Model file for the job. Use its own axes, mm. Face numbers are marked on the shaded views. A direction names the side the tool comes from. Round coordinates to 2 decimals unless told otherwise and drop trailing zeros. Loops run counter-clockwise (first coordinate to the right, second up) from the corner with the lowest first, then second, coordinate; pieces in that order, holes last. Notation, with made-up numbers: M -38.5,-22.75 L -27.5,-22.75 A32 cw -27.5,13.25 Z; hole C 87.5,40 d3. An arc over 180 degrees is marked long. Answer in a Markdown table with one row per item.
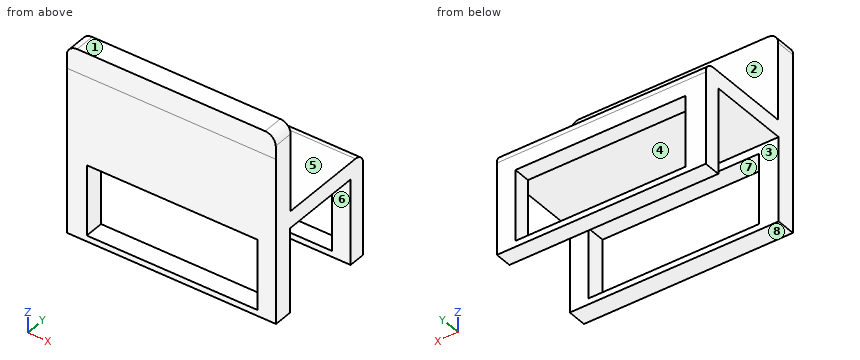
from build123d import *

# Parameters (mm, degrees)
F1_DEPTH = 101.6
F2_R     = 5.08
F4_W     = 83.005025
F4_H     = 34.228876
F5_DEPTH = 25.4
F3_W     = 82.719785
F3_H     = 34.51412
F6_DEPTH = 25.4


with BuildPart() as f1:
    # F0 (on Right) → F1 (new body)
    with BuildSketch(Plane.YZ):
        Polygon((-64.356416, 42.612657), (-64.071178, 30.91779), (-64.071178, -49.234834), (-54.658234, -49.234834), (-54.658234, -8.160179), (-14.724543, -8.160179), (-14.724543, -49.805317), (-6.452564, -49.805317), (-6.452564, -7.589698), (-6.452564, 0), (-54.372992, 0), (-54.372992, 42.612657), align=None)
    extrude(amount=F1_DEPTH)

    # F2
    f2_edges = [f1.edges().sort_by_distance(p)[0] for p in [
        (101.6, -59.364704, 42.612657),
        (0, -59.364704, 42.612657),
        (50.8, -6.452564, 0),
    ]]
    fillet(f2_edges, radius=F2_R)

    # F4 (on face) → F5 (cut)
    with BuildSketch(Plane.XZ.offset(64.071178)):
        with Locations((51.064864, -29.237166)):
            Rectangle(F4_W, F4_H)
    extrude(amount=-F5_DEPTH, mode=Mode.SUBTRACT)

    # F3 (on face) → F6 (cut)
    with BuildSketch(Plane(origin=(0, -6.452564, 0), x_dir=(-1, 0, 0), z_dir=(0, 1, 0))):
        with Locations((-51.207484, -29.665028)):
            Rectangle(F3_W, F3_H)
    extrude(amount=-F6_DEPTH, mode=Mode.SUBTRACT)


solid = f1.part
1. Saw through at A-A (x = 62). Write the cut outline in (y, z), and give its area (3 significant figures).
Verdict:
| item | result |
|---|---|
| outline | M -64.36,42.61 L -64.07,30.92 L -64.07,-12.12 L -54.66,-12.12 L -54.66,-8.16 L -14.72,-8.16 L -14.72,-12.41 L -6.45,-12.41 L -6.45,-5.08 A5.08 ccw -11.53,0 L -54.37,0 L -54.37,42.61 Z; M -64.07,-49.23 L -54.66,-49.23 L -54.66,-46.35 L -64.07,-46.35 Z; M -14.72,-49.81 L -6.45,-49.81 L -6.45,-46.92 L -14.72,-46.92 Z |
| area | 1,000 mm² |
2. Saw through at D-D (y = -13.5). Write the cut outline in (x, z), and give its area (3 significant figures).
Verdict:
| item | result |
|---|---|
| outline | M 0,-49.81 L 101.6,-49.81 L 101.6,0 L 0,0 Z; hole M 9.85,-46.92 L 92.57,-46.92 L 92.57,-12.41 L 9.85,-12.41 Z |
| area | 2,210 mm² |
3. Saw through at B-B (z = -30.5). Write the cut outline in (x, y), and give its area (3 significant figures).
Verdict:
| item | result |
|---|---|
| outline | M 0,-64.07 L 9.56,-64.07 L 9.56,-54.66 L 0,-54.66 Z; M 0,-14.72 L 9.85,-14.72 L 9.85,-6.45 L 0,-6.45 Z; M 92.57,-64.07 L 101.6,-64.07 L 101.6,-54.66 L 92.57,-54.66 Z; M 92.57,-14.72 L 101.6,-14.72 L 101.6,-6.45 L 92.57,-6.45 Z |
| area | 331 mm² |
4. Pin check, flat tips, straight feed: pin 1 (3 mm diameter, centred on y = -57, z = -30.5, fed in from -X); pin 2 (1.5 mm diameter, centred on x = 12.5, z = -13, fed in from -Y); pin 3 (6.5 mm diameter, centred on x = 40.5, y = -9, fed in from +Z); pin 4 (7.5 mm diameter, centred on x = 50.5, y = -59, fed in from -Z). Stop position of each tip, or through.
Verdict:
| item | result |
|---|---|
| pin 1 | stops at x = 0 |
| pin 2 | stops at y = -14.72 |
| pin 3 | stops at z = 0 |
| pin 4 | stops at z = -49.23 |
5. Wall check: probe 1 along Y at (x, z) = (57, -12); probe 2 along X at (y, z) = (-57, -38); probe 3 along Z at (x, y) = (85, -57). Give the ranges that are in metal, low to high.
Verdict:
| item | result |
|---|---|
| probe 1 | y = -64.07 to -54.66, -14.72 to -6.45 |
| probe 2 | x = 0 to 9.56, 92.57 to 101.6 |
| probe 3 | z = -49.23 to -46.35, -12.12 to 42.61 |
6. Tool access for the marked faces 5, 6, 7 and 8: list every direction of +Z, -Z, +X, -X, +Y, -Y with a clear straight run to the whole face (end or side of a thin tool).
Verdict:
| item | result |
|---|---|
| face 5 | +Z, +X, -X, +Y |
| face 6 | -Z, +X, -X |
| face 7 | -Y |
| face 8 | -Z, +X, -X, -Y |
7. Saw through at C-C (y = -57.5). Write the cut outline in (x, z).
Verdict:
| item | result |
|---|---|
| outline | M 0,-49.23 L 101.6,-49.23 L 101.6,37.53 A5.08 ccw 96.52,42.61 L 5.08,42.61 A5.08 ccw 0,37.53 Z; hole M 9.56,-46.35 L 92.57,-46.35 L 92.57,-12.12 L 9.56,-12.12 Z |
8. Mould opens along Y. For the marked faces 1, 2, 3 and 4 say: +Y half, -Y half, draft (parallel to the pull), parting line (faces both ways), or undercut.
Verdict:
| item | result |
|---|---|
| face 1 | draft |
| face 2 | +Y half |
| face 3 | undercut |
| face 4 | undercut |
